```python
from build123d import *

# Parameters (mm, degrees)
CYLINDER016017_R            = 1.45
CYLINDER016017_DEPTH        = 10
CYLINDER016015_R            = 3.1
CYLINDER016015_DEPTH        = 10
CYLINDER016016_R            = 3.1
CYLINDER016016_DEPTH        = 10
BOX021_W                    = 7.8
BOX021_H                    = 7.5
BOX021_DEPTH                = 20
BOX022_W                    = 16
BOX022_H                    = 6
BOX022_DEPTH                = 20
CHAMFER016016008004002_SIZE = 3


with BuildPart() as cylinder033:
    # Cylinder016017 → Cylinder016017 (new body)
    with BuildSketch(Plane(origin=(0, 0.5, 10), x_dir=(1, 0, 0), z_dir=(0, 1, 0))):
        Circle(CYLINDER016017_R)
    extrude(amount=CYLINDER016017_DEPTH)


with BuildPart() as cylinder031:
    # Cylinder016015 → Cylinder016015 (new body)
    with BuildSketch(Plane(origin=(0, 0.5, 4), x_dir=(1, 0, 0), z_dir=(0, 1, 0))):
        Circle(CYLINDER016015_R)
    extrude(amount=CYLINDER016015_DEPTH)


with BuildPart() as fusion018004:
    # Cylinder016016 → Cylinder016016 (new body)
    with BuildSketch(Plane(origin=(0, 0.5, 16), x_dir=(1, 0, 0), z_dir=(0, 1, 0))):
        Circle(CYLINDER016016_R)
    extrude(amount=CYLINDER016016_DEPTH)

    # Fusion018004: union Cylinder031
    add(cylinder031.part)


with BuildPart() as fusion018004_1:
    # Fusion018004 placement: moved
    add(fusion018004.part.moved(Location((0, 1, 0))))


with BuildPart() as cube021:
    # Box021 → Box021 (new body)
    with BuildSketch(Plane(origin=(-3.9, 0.5, 0), x_dir=(1, 0, 0), z_dir=(0, 0, 1))):
        with Locations((3.9, 3.75)):
            Rectangle(BOX021_W, BOX021_H)
    extrude(amount=BOX021_DEPTH)


with BuildPart() as magnet_nut:
    # Box022 → Box022 (new body)
    with BuildSketch(Plane(origin=(-8, 2, 0), x_dir=(1, 0, 0), z_dir=(0, 0, 1))):
        with Locations((8, 3)):
            Rectangle(BOX022_W, BOX022_H)
    extrude(amount=BOX022_DEPTH)

    # Chamfer016016008004002
    chamfer016016008004002_edges = [magnet_nut.edges().sort_by_distance(p)[0] for p in [
        (-8, 8, 10),
        (8, 8, 10),
    ]]
    chamfer(chamfer016016008004002_edges, length=CHAMFER016016008004002_SIZE)

    # Fusion018005: union Cube021
    add(cube021.part)

    # Cut010011008008: cut Fusion018004
    add(fusion018004_1.part, mode=Mode.SUBTRACT)

    # Cut010011008009: cut Cylinder033
    add(cylinder033.part, mode=Mode.SUBTRACT)


solid = magnet_nut.part
```
The model under review builds one solid part; all positions refer to its coordinate system, in mm. A direction names the side the tool comes from. Round coordinates to 2 decimals unless told otherwise and drop trailing zeros. Order: outer loops, then holes, each group sorted by start corner. A loop starts at its lowest first (then second) coordinate and runs counter-clockwise, first axis right, second up. Notation, with made-up numbers: M 85,6 L 128,6 A34 cw 128,45 Z; hole C 28,-23.75 d5. An arc over 180 degrees is marked long. Use a Markdown table: item, result.
1) Draft analysis for pull direction X (two halves, no side actions). For faces 6 (the face through (6, 2, 10)), 7 (the face through (8, 3, 10)), 8 (the face through (0, 1.5, 4)), state which applies: released by +X, released by -X, zero draft, split by the parting line, or undercut.
Report:
| item | result |
|---|---|
| face 6 | zero draft |
| face 7 | released by +X |
| face 8 | undercut |
2) Consider section A-A (x = 0). Write out the cut boundary in (y, z), then the cut area to 4 significant figures.
Report:
| item | result |
|---|---|
| outline | M 0.5,0 L 8,0 L 8,0.9 L 1.5,0.9 L 1.5,7.1 L 8,7.1 L 8,8.55 L 0.5,8.55 Z; M 0.5,11.45 L 8,11.45 L 8,12.9 L 1.5,12.9 L 1.5,19.1 L 8,19.1 L 8,20 L 0.5,20 Z |
| area | 47.65 mm^2 |
3) Tool access review of faces 1 (the face through (3.9, 1, 10)), 2 (the face through (-6, 2, 10)), 3 (the face through (0, 1.5, 16)), 4 (the face through (-0.314, 4.198, 11.416)), 5 (the face through (6, 7, 10)): name each direction out of +Z, -Z, +X, -X, +Y, -Y from which nothing blocks a thin tool from reaching the whole face with its end or side.
Report:
| item | result |
|---|---|
| face 1 | +Z, -Z, +X, -Y |
| face 2 | +Z, -Z, -X, -Y |
| face 3 | +Y |
| face 4 | +Y, -Y |
| face 5 | +Z, -Z, +X, +Y |
4) Consider section C-C (z = 10). Write out the cut boundary in (x, y).
Report:
| item | result |
|---|---|
| outline | M -8,2 L -3.9,2 L -3.9,0.5 L -1.45,0.5 L -1.45,8 L -5,8 L -8,5 Z; M 1.45,0.5 L 3.9,0.5 L 3.9,2 L 8,2 L 8,5 L 5,8 L 1.45,8 Z |
5) Consider section B-B (y = 6.25). Write out the cut boundary in (x, z).
Report:
| item | result |
|---|---|
| outline | M -6.75,0 L 6.75,0 L 6.75,20 L -6.75,20 Z; hole C 0,4 d6.2; hole C 0,16 d6.2; hole C 0,10 d2.9 |
6) Consider section D-D (z = 16). Write out the cut boundary in (x, y).
Report:
| item | result |
|---|---|
| outline | M -8,2 L -3.9,2 L -3.9,0.5 L 3.9,0.5 L 3.9,2 L 8,2 L 8,5 L 5,8 L 3.1,8 L 3.1,1.5 L -3.1,1.5 L -3.1,8 L -5,8 L -8,5 Z |
7) Wall thickness on line 1 along Z through (x, y) = (0, 5.5); line 2 along X through (y, z) = (2.5, 10); line 3 along Z through (x, y) = (-2.5, 2.5): over which ranges is each line inside the solid? List them lowest first. Write a range as [from, to].
Report:
| item | result |
|---|---|
| line 1 | [0, 0.9], [7.1, 8.55], [11.45, 12.9], [19.1, 20] |
| line 2 | [-8, -1.45], [1.45, 8] |
| line 3 | [0, 2.17], [5.83, 14.17], [17.83, 20] |
8) Insertion check: pin 1 (3.5 mm diameter, centred on x = 0, z = 16, fed in from +Y); pin 2 (1.7 mm diameter, centred on x = 0, z = 10, fed in from +Y); pin 3 (1 mm diameter, centred on y = 6, z = 10, fed in from -X); pin 4 (1.6 mm diameter, centred on y = 1, z = 10, fed in from +X). Each pin has a flat end and moves straight along its axis. Give the tip position at first contact, or say it passes through.
Report:
| item | result |
|---|---|
| pin 1 | y = 1.5 |
| pin 2 | through |
| pin 3 | x = -7.5 |
| pin 4 | x = 3.9 |
